Can you work these out from the model? Positions are in its coordinate system, mm. Give positions to 0.01 mm unless a question says otherwise; leave off trailing zeros. Write each loop counter-clockwise with the first axis right and the second up, starting at its lowest first coordinate (ties: lowest second). Pieces come first, ordered by that corner, then holes.
from build123d import *

# Parameters (mm, degrees)
F0_R     = 2
F1_DEPTH = 10
F2_R     = 2
F3_DEPTH = 25


# Not quite as in the source:
# - a feature names something its author has since deleted; it is built from what else it names


with BuildPart() as f1:
    # F0 (on Top) → F1 (new body)
    with BuildSketch(Plane.XY):
        with BuildLine():
            Line((-3.5, 15), (-3.5, 0))
            ThreePointArc((-3.5, 0), (0, -3.5), (3.5, 0))
            Line((3.5, 0), (3.5, 15))
            Line((3.5, 15), (-3.5, 15))
        make_face()
        Circle(F0_R, mode=Mode.SUBTRACT)
    extrude(amount=F1_DEPTH)

    # F2 (on face) → F3 (cut)
    with BuildSketch(Plane.YZ.offset(3.5)):
        with Locations((11.6752159595, 5)):
            Circle(F2_R)
        with BuildLine():
            ThreePointArc((14.028986054, 7.5826258022), (14.7403982458, 6.8530370755), (15, 5.8676366767))
            Line((15, 5.8676366767), (15, 10))
            Line((15, 10), (10, 10))
            Line((10, 10), (14.028986054, 7.5826258022))
        make_face()
    extrude(amount=-F3_DEPTH, mode=Mode.SUBTRACT)


solid = f1.part
(1) If we mould it in two halves opening along Y, with no side actions, what happens to faces 1 (the face through (0, -2, 5)), 2 (the face through (-0.1, -3.5, 4.9)), 3 (the face through (0, 12, 8.8)), 4 (the face through (0, 6, 0))? For each: +Y half, -Y half, draft (parallel to the pull), parting line (faces both ways), or undercut.
Returned:
face 1: undercut
face 2: -Y half
face 3: +Y half
face 4: draft
(2) If I drill on L1, parallel to Y at x = 0.25, z = 4.25; L2, parallel to Y at x = 1.25, z = 5.75; L3, parallel to Y at x = -0.75, z = 7.25, over which ranges is the centre line in solid material (lowest first)?
Returned:
L1: y = -3.49 to -1.98, 1.98 to 9.82, 13.53 to 15
L2: y = -3.27 to -1.56, 1.56 to 9.82, 13.53 to 15
L3: y = -3.42 to -1.85, 1.85 to 14.45
(3) Imagine slicing it at C-C, the plane y = -0.75. Write out the boundary of the cut face in (x, z).
Returned:
outline: (-3.42, 0) - (-1.85, 0) - (-1.85, 10) - (-3.42, 10) - close; (1.85, 0) - (3.42, 0) - (3.42, 10) - (1.85, 10) - close
(4) Imagine slicing it at D-D, the plane z = 3.25. Write out the boundary of the cut face in (x, y).
Returned:
outline: (-3.5, 0) arc R3.5 ccw to (3.5, 0) - (3.5, 10.71) - (-3.5, 10.71) - close; (-3.5, 12.64) - (3.5, 12.64) - (3.5, 15) - (-3.5, 15) - close; hole circle Ø4 at (0, 0)
(5) Will these pins go through, and if not, where does the flat tip stop? P1, Ø2.5, axis at y = 11.68, z = 5, coming from the -X side; P2, Ø1.5, axis at x = -1.5, y = -0.5, coming from the -Z side; P3, Ø1.5, axis at x = 1.5, z = 8, coming from the +Y side.
Returned:
P1: passes through
P2: stops at z = 0
P3: stops at y = 14.45
(6) Imagine slicing it at B-B, the plane z = 5. Write out the boundary of the cut face in (x, y).
Returned:
outline: (-3.5, 0) arc R3.5 ccw to (3.5, 0) - (3.5, 9.68) - (-3.5, 9.68) - close; (-3.5, 13.68) - (3.5, 13.68) - (3.5, 15) - (-3.5, 15) - close; hole circle Ø4 at (0, 0)
(7) Imagine slicing it at A-A, the plane x = 0. Write out the boundary of the cut face in (y, z), plus the area to 3 significant figures.
Returned:
outline: (-3.5, 0) - (-2, 0) - (-2, 10) - (-3.5, 10) - close; (2, 0) - (15, 0) - (15, 5.87) arc R2 ccw to (14.03, 7.58) - (10, 10) - (2, 10) - close; hole circle Ø4 at (11.68, 5)
area: 125 mm2
